For this review, take the finished solid that the model builds, in its own axes (mm). A direction names the side the tool comes from. Coordinates: 2 decimals unless noted, no trailing zeros. Order: outer loops, then holes, each group sorted by start corner. A loop starts at its lowest first (then second) coordinate and runs counter-clockwise, first axis right, second up. Notation, with made-up numbers: (62, 10) -> (90, 10) arc R16 cw to (90, 23) -> close; hole circle Ø3 at (12.5, 42). An arc over 180 degrees is marked (long way). Answer as a JSON object with one key per item and string values. Group by question number.
1) Add section C-C, the plane z = 46. Write out the cut boundary in (x, y).
2) Add section D-D, the plane x = 102. Write out the cut boundary in (y, z), then the cut area to 3 significant figures.
3) For pin 1 (12 mm diameter, centred on x = -65, y = 89.5, fed in from -Z); pin 2 (6 mm diameter, centred on y = 49, z = 184, fed in from -X); pin 3 (1.5 mm diameter, centred on x = -70.5, y = 150.5, fed in from -Z), all flat-tipped, find the tip position at first contact; note any pin that passes through.
4) Add section B-B, the plane x = 0. Write out the cut boundary in (y, z), then the cut area to 3 significant figures.
5) Machinability: for faces 1 (the flat face through (0, 90, -97)), 2 (the flat face through (35.702, 159.507, 148.396)), 3 (the flat face through (-160.063, 144.79, 68.785)), which of the approach directions +Z, -Z, +X, -X, +Y, -Y give a long, thin tool a straight path to every point of the face, cutting with its end or side? Answer none if there is none.
6) Add section A-A, the plane y = 143.5. Write out the cut boundary in (x, z).
7) Wall thickness on L1, parallel to Z at x = 0, y = 112; L2, parallel to Y at x = -144, z = 0; L3, parallel to Z at x = 23.5, y = 97.5: over which ranges is each line inside the solid? List them lowest first.
8) Draft analysis for pull direction Z (two halves, no side actions). For faces 4 (the cylindrical face through (-2.93, 164.93, 219.04)), 5 (the cylindrical face through (2.86, 83.81, 239.98)), 6 (the flat face through (64.126, 159.507, 176.866)), state which applies: +Z half, -Z half, draft (parallel to the pull), parting line (faces both ways), or undercut.
from build123d import *

# Parameters (mm, degrees)
BOSS_EXTRUDE1_DEPTH = 130
BOSS_EXTRUDE2_DEPTH = 40
SKETCH4_R           = 35
CUT_EXTRUDE1_DEPTH  = 40
BOSS_EXTRUDE3_DEPTH = 30
CUT_EXTRUDE2_DEPTH  = 1
CIRPATTERN1_COUNT   = 4
CIRPATTERN1_ANGLE   = 60


with BuildPart() as part:
    # Sketch2 → Boss-Extrude1 (new body)
    with BuildSketch(Plane(origin=(0, 0, 0), x_dir=(1, 0, 0), z_dir=(0, 1, 0))):
        with BuildLine():
            Line((-172, 150), (-175, -150))
            ThreePointArc((-175, -150), (0, -240), (175, -150))
            Line((175, -150), (172, 150))
            ThreePointArc((172, 150), (0, 276.934003354), (-172, 150))
        make_face()
    extrude(amount=BOSS_EXTRUDE1_DEPTH)

    # Sketch3 → Boss-Extrude2 (add)
    with BuildSketch(Plane(origin=(0, 130, 0), x_dir=(1, 0, 0), z_dir=(0, 1, 0))):
        with BuildLine():
            Line((-175, -150), (-174.71, -121))
            ThreePointArc((-174.71, -121), (0, -219.05898872), (174.71, -121))
            Line((174.71, -121), (175, -150))
            ThreePointArc((175, -150), (0, -240), (-175, -150))
        make_face()
    extrude(amount=BOSS_EXTRUDE2_DEPTH)

    # Sketch4 → Cut-Extrude1 (cut)
    with BuildSketch(Plane(origin=(0, 130, 0), x_dir=(1, 0, 0), z_dir=(0, 1, 0))):
        with Locations((0, 96.934003354)):
            Circle(SKETCH4_R)
    extrude(amount=-CUT_EXTRUDE1_DEPTH, mode=Mode.SUBTRACT)

    # Sketch5 → Boss-Extrude3 (add)
    with BuildSketch(Plane(origin=(0, 130, 0), x_dir=(1, 0, 0), z_dir=(0, 1, 0))):
        with BuildLine():
            Line((-174.71, -121), (-145, -15.088169216))
            ThreePointArc((-145, -15.088169216), (0, -117.466388714), (145, -15.088169216))
            Line((145, -15.088169216), (174.71, -121))
            ThreePointArc((174.71, -121), (0, -219.05898872), (-174.71, -121))
        make_face()
    extrude(amount=BOSS_EXTRUDE3_DEPTH)

    # Sketch6 → Cut-Extrude2 (cut)
    with BuildSketch(Plane(origin=(0, 160, 0), x_dir=(1, 0, 0), z_dir=(0, 1, 0))):
        Polygon((169.306747394, -126.764048286), (119.216917014, -60.582412673), (88.83715416, -83.575455293), (138.92698454, -149.757090907), align=None)
    cut_extrude2 = extrude(amount=-CUT_EXTRUDE2_DEPTH, mode=Mode.SUBTRACT)

    # CirPattern1: Cut-Extrude2 ×4 about axis
    cirpattern1_axis = Axis((0, 0, -96.934003354), (0, -1, 0))
    for i in range(1, CIRPATTERN1_COUNT):
        add(cut_extrude2.rotate(cirpattern1_axis, i * CIRPATTERN1_ANGLE / (CIRPATTERN1_COUNT - 1)), mode=Mode.SUBTRACT)


solid = part.part
Output values:
{
 "1": {"outline": "(-173.96, 0) -> (173.96, 0) -> (173.96, 130) -> (153.67, 130) -> (153.67, 160) -> (129.95, 160) -> (129.95, 130) -> (-129.95, 130) -> (-129.95, 160) -> (-153.67, 160) -> (-153.67, 130) -> (-173.96, 130) -> close"},
 "2": {"outline": "(0, -245.24) -> (130, -245.24) -> (130, 78.8) -> (159, 78.8) -> (159, 100.97) -> (160, 100.97) -> (160, 191.83) -> (170, 191.83) -> (170, 214.28) -> (0, 214.28) -> close", "area": "64,000 mm²"},
 "3": {"pin 1": "stops at z = -266.99", "pin 2": "stops at x = -148", "pin 3": "stops at z = 99.98"},
 "4": {"outline": "(0, -276.93) -> (130, -276.93) -> (130, -131.93) -> (90, -131.93) -> (90, -61.93) -> (130, -61.93) -> (130, 117.47) -> (160, 117.47) -> (160, 219.06) -> (170, 219.06) -> (170, 240) -> (0, 240) -> close", "area": "68,300 mm²"},
 "5": {"face 1": "+Y", "face 2": "-Z, +Y", "face 3": "-Z, -X, +Y"},
 "6": {"outline": "(-175, 150) -> (-174.71, 121) -> (-145, 15.09) arc R153.87 cw to (145, 15.09) -> (174.71, 121) -> (175, 150) arc R215.14 ccw to start"},
 "7": {"L1": "z = -276.93 to -131.93, -61.93 to 240", "L2": "y = 0 to 130", "L3": "z = -275.39 to -122.87, -71 to 238.71"},
 "8": {"face 4": "-Z half", "face 5": "+Z half", "face 6": "undercut"}
}
